Source: CAD feature listing. Evaluate the final solid. Frame: model axes, mm. Face numbers are marked on the shaded views. A direction names the side the tool comes from. Give positions to 0.01 mm unless a question says otherwise; leave off trailing zeros. Loops run counter-clockwise (first coordinate to the right, second up) from the corner with the lowest first, then second, coordinate; pieces in that order, holes last. Notation, with made-up numbers: M -35.5,41 L -4.5,41 A20 cw -4.5,63 Z; hole C -33.5,-21.5 d5. An arc over 180 degrees is marked long. Answer in a Markdown table with one row per item.
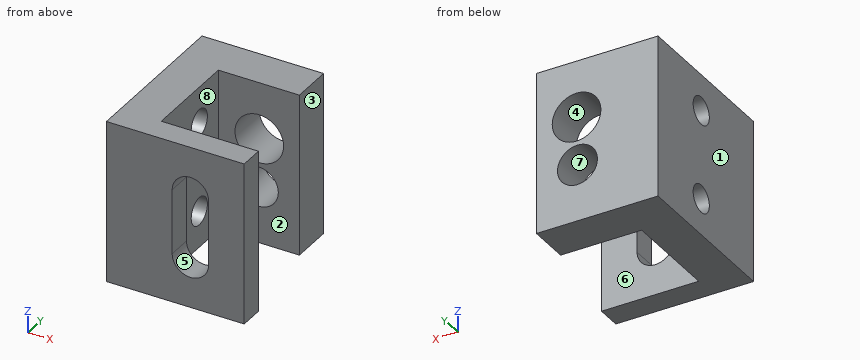
```python
from build123d import *

# Parameters (mm, degrees)
SKETCH1_W            = 15
SKETCH1_H            = 20
BOSS_EXTRUDE1_DEPTH  = 5.08
SKETCH2_W            = 5
SKETCH2_H            = 20
BOSS_EXTRUDE2_DEPTH  = 15
M3_CLEARANCE_HOLE1_D = 3.4
SKETCH7_W            = 20
SKETCH7_H            = 3
BOSS_EXTRUDE3_DEPTH  = 12
SKETCH3_R            = 2.4638
CUT_EXTRUDE1_DEPTH   = 12
SKETCH4_R            = 3
CUT_EXTRUDE2_DEPTH   = 12
CUT_EXTRUDE3_DEPTH   = 12


with BuildPart() as part:
    # Sketch1 → Boss-Extrude1 (new body)
    with BuildSketch(Plane(origin=(0, 0, 0), x_dir=(1, 0, 0), z_dir=(0, 1, 0))):
        Rectangle(SKETCH1_W, SKETCH1_H)
    extrude(amount=BOSS_EXTRUDE1_DEPTH)

    # Sketch2 → Boss-Extrude2 (add)
    with BuildSketch(Plane(origin=(0, 0, 0), x_dir=(-1, 0, 0), z_dir=(0, -1, 0))):
        with Locations((5, 0)):
            Rectangle(SKETCH2_W, SKETCH2_H)
    extrude(amount=BOSS_EXTRUDE2_DEPTH)

    # M3 Clearance Hole1 (through all)
    with Locations(Plane(origin=(-2.5, 0, 0), x_dir=(0, 0, -1), z_dir=(1, 0, 0))):
        with Locations((5.5, -4), (-5.5, -4)):
            Hole(M3_CLEARANCE_HOLE1_D / 2)

    # Sketch7 → Boss-Extrude3 (add)
    with BuildSketch(Plane(origin=(-2.5, 0, 0), x_dir=(0, 0, -1), z_dir=(1, 0, 0))):
        with Locations((0, -13.5)):
            Rectangle(SKETCH7_W, SKETCH7_H)
    extrude(amount=BOSS_EXTRUDE3_DEPTH)

    # Sketch3 → Cut-Extrude1 (cut)
    with BuildSketch(Plane(origin=(0, 5.08, 0), x_dir=(1, 0, 0), z_dir=(0, 1, 0))):
        with Locations((2.435150465, 3)):
            Circle(SKETCH3_R)
    extrude(amount=-CUT_EXTRUDE1_DEPTH, mode=Mode.SUBTRACT)

    # Sketch4 → Cut-Extrude2 (cut)
    with BuildSketch(Plane(origin=(0, 5.08, 0), x_dir=(1, 0, 0), z_dir=(0, 1, 0))):
        with Locations((2.551153976, -3)):
            Circle(SKETCH4_R)
    extrude(amount=-CUT_EXTRUDE2_DEPTH, mode=Mode.SUBTRACT)

    # Sketch8 → Cut-Extrude3 (cut)
    with BuildSketch(Plane(origin=(0, -15, 0), x_dir=(-1, 0, 0), z_dir=(0, -1, 0))):
        with BuildLine():
            Line((-0.611529575, 4), (-0.611529575, -4))
            ThreePointArc((-0.611529575, -4), (-2.861529575, -6.25), (-5.111529575, -4))
            Line((-5.111529575, -4), (-5.111529575, 4))
            ThreePointArc((-5.111529575, 4), (-2.861529575, 6.25), (-0.611529575, 4))
        make_face()
    extrude(amount=-CUT_EXTRUDE3_DEPTH, mode=Mode.SUBTRACT)


solid = part.part
```
1) Section C-C, the plane y = -13.5. Return loops of the section in (x, z), then the cut area to 3 significant figures.
Reply:
| item | result |
|---|---|
| outline | M -7.5,-10 L 9.5,-10 L 9.5,10 L -7.5,10 Z; hole M 0.61,-4 A2.25 ccw 5.11,-4 L 5.11,4 A2.25 ccw 0.61,4 Z |
| area | 288 mm² |
2) Section B-B, the plane z = 3. Return loops of the section in (x, y).
Reply:
| item | result |
|---|---|
| outline | M -7.5,-15 L 0.61,-15 L 0.61,-12 L -2.5,-12 L -2.5,0 L -0.45,0 L -0.45,5.08 L -7.5,5.08 Z; M 5.11,-15 L 9.5,-15 L 9.5,-12 L 5.11,-12 Z; M 5.55,0 L 7.5,0 L 7.5,5.08 L 5.55,5.08 Z |
3) Pull-direction query (X, two-part tool) for the marked faces 5, 6, 7 and 8; classes: released by +X, released by -X, zero draft, split by the parting line, or undercut.
Reply:
| item | result |
|---|---|
| face 5 | undercut |
| face 6 | zero draft |
| face 7 | undercut |
| face 8 | released by +X |
4) Section A-A, the plane y = -4. Return loops of the section in (x, z), then the cut area to 3 significant figures.
Reply:
| item | result |
|---|---|
| outline | M -7.5,-10 L -2.5,-10 L -2.5,-7.2 L -7.5,-7.2 Z; M -7.5,-3.8 L -2.5,-3.8 L -2.5,3.8 L -7.5,3.8 Z; M -7.5,7.2 L -2.5,7.2 L -2.5,10 L -7.5,10 Z |
| area | 66.0 mm² |
5) Set-up query: the marked faces 1, 2, 3 and 4. Return all of +Z, -Z, +X, -X, +Y, -Y with unobstructed straight access to the full face (end or side cutting, diameter ignored); none if empty.
Reply:
| item | result |
|---|---|
| face 1 | +Z, -Z, -X, +Y, -Y |
| face 2 | +Z, -Z, +X |
| face 3 | +Z, -Z, +X, +Y |
| face 4 | +Y |
6) Section D-D, the plane x = 4. Return loops of the section in (y, z), then the cut area to 3 significant figures.
Reply:
| item | result |
|---|---|
| outline | M -15,-10 L -12,-10 L -12,-5.94 L -15,-5.94 Z; M -15,5.94 L -12,5.94 L -12,10 L -15,10 Z; M 0,-10 L 5.08,-10 L 5.08,-4.9 L 0,-4.9 Z; M 0,-1.1 L 5.08,-1.1 L 5.08,0.37 L 0,0.37 Z; M 0,5.63 L 5.08,5.63 L 5.08,10 L 0,10 Z |
| area | 79.9 mm² |
7) Pin query (flat end, axial travel): pin 1 Ø4 at (y, z) = (2.5, 2) entering from +X; pin 2 Ø5.5 at (y, z) = (-4, 5.5) entering from +X. Return the tip coordinate at first contact, or that it passes through.
Reply:
| item | result |
|---|---|
| pin 1 | stops at x = 7.5 |
| pin 2 | stops at x = -2.5 |
8) Material intervals for L1, parallel to Y at x = 7.25, z = 4; L2, parallel to Z at x = 0.75, y = 3.75; L3, parallel to Z at x = 2.75, y = 2.75, sorted ascending.
Reply:
| item | result |
|---|---|
| L1 | y = -15 to -12, 0 to 5.08 |
| L2 | z = -10 to -4.8, -1.2 to 0.6, 5.4 to 10 |
| L3 | z = -10 to -5.44, -0.56 to 0.01, 5.99 to 10 |
